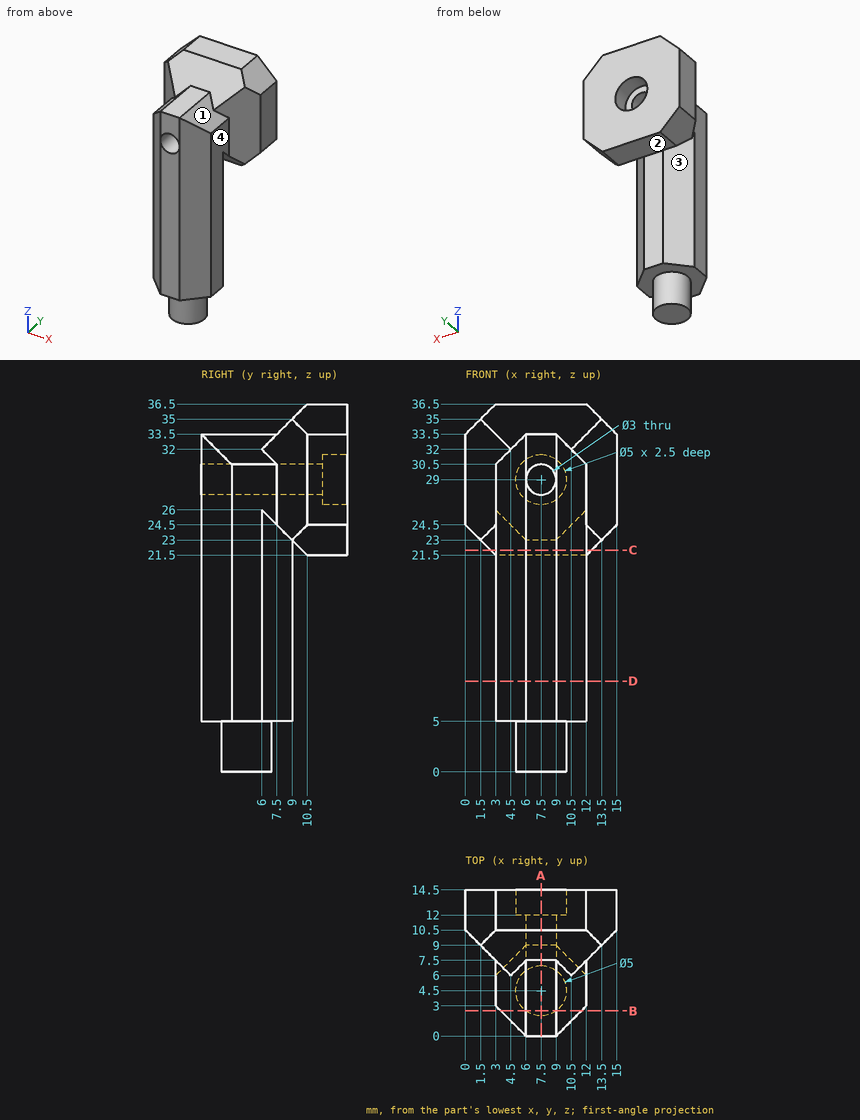
Input: dimensioned drawing with shaded views. Units: mm. Origin: part minimum x, y, z. A direction names the side the tool comes from. Coordinates: 2 decimals unless noted, no trailing zeros. Loops run counter-clockwise (first coordinate to the right, second up) from the corner with the lowest first, then second, coordinate; pieces in that order, holes last. Notation, with made-up numbers: M 10.25,30 L 51.25,30 A27 cw 51.25,53 Z; hole C 85.25,53.5 d6. An arc over 180 degrees is marked long. One line per item, written item: value. Start each with the question number.
1) Material intervals for L1, parallel to X at y = 12.75, z = 29; L2, parallel to X at y = 3.5, z = 29; L3, parallel to Z at x = 4, y = 2.75, sorted ascending. Write a range as from..to.
2) Cut plane C-C (z = 22). Return loops of the section in (x, y).
3) Pin query (flat end, axial travel): P1, Ø2.5, axis at x = 7.5, z = 29, coming from the -Y side; P2, Ø3.5, axis at x = 7, z = 18, coming from the +Y side; P3, Ø4, axis at x = 12.5, z = 27, coming from the -Y side; P4, Ø0.9, axis at x = 7.5, y = 3.5, coming from the +Z side. Return the tip coordinate at first contact, or that it passes through.
4) Cut plane B-B (y = 2.5). Return loops of the section in (x, z).
5) Cut plane A-A (x = 7.5). Return loops of the section in (y, z), then the cut area to 3 significant figures.
6) Reachability of the marked faces 1, 2, 3 and 4 from +Z, -Z, +X, -X, +Y, -Y: full face, straight path, thin tool, end or side. Return the list, or none.
7) Cut plane D-D (z = 9). Return loops of the section in (x, y).
Evaluation:
1. L1: 0..5, 10..15
1. L2: 3..6, 9..12
1. L3: 5..31.5
2. outline: M 2.5,10 L 12.5,10 L 12.5,14.5 L 2.5,14.5 Z; M 3,3 L 6,0 L 9,0 L 12,3 L 12,6 L 9,9 L 6,9 L 3,6 Z
3. P1: through
3. P2: y = 9
3. P3: y = 1.5
3. P4: z = 33.5
4. outline: M 3.5,5 L 6,5 L 6,0 L 9,0 L 9,5 L 11.5,5 L 11.5,31 L 9,33.5 L 6,33.5 L 3.5,31 Z; hole C 7.5,29 d3
5. outline: M 0,5 L 2,5 L 2,0 L 7,0 L 7,5 L 9,5 L 9,23 L 10.5,21.5 L 14.5,21.5 L 14.5,26.5 L 12,26.5 L 12,27.5 L 0,27.5 Z; M 0,30.5 L 12,30.5 L 12,31.5 L 14.5,31.5 L 14.5,36.5 L 10.5,36.5 L 7.5,33.5 L 0,33.5 Z
5. area: 314 mm^2
6. face 1: +Z, +X, -Y
6. face 2: -Z, +X, -X, +Y
6. face 3: -Z, -X
6. face 4: +Z, -Z, +X, -Y
7. outline: M 3,3 L 6,0 L 9,0 L 12,3 L 12,6 L 9,9 L 6,9 L 3,6 Z
